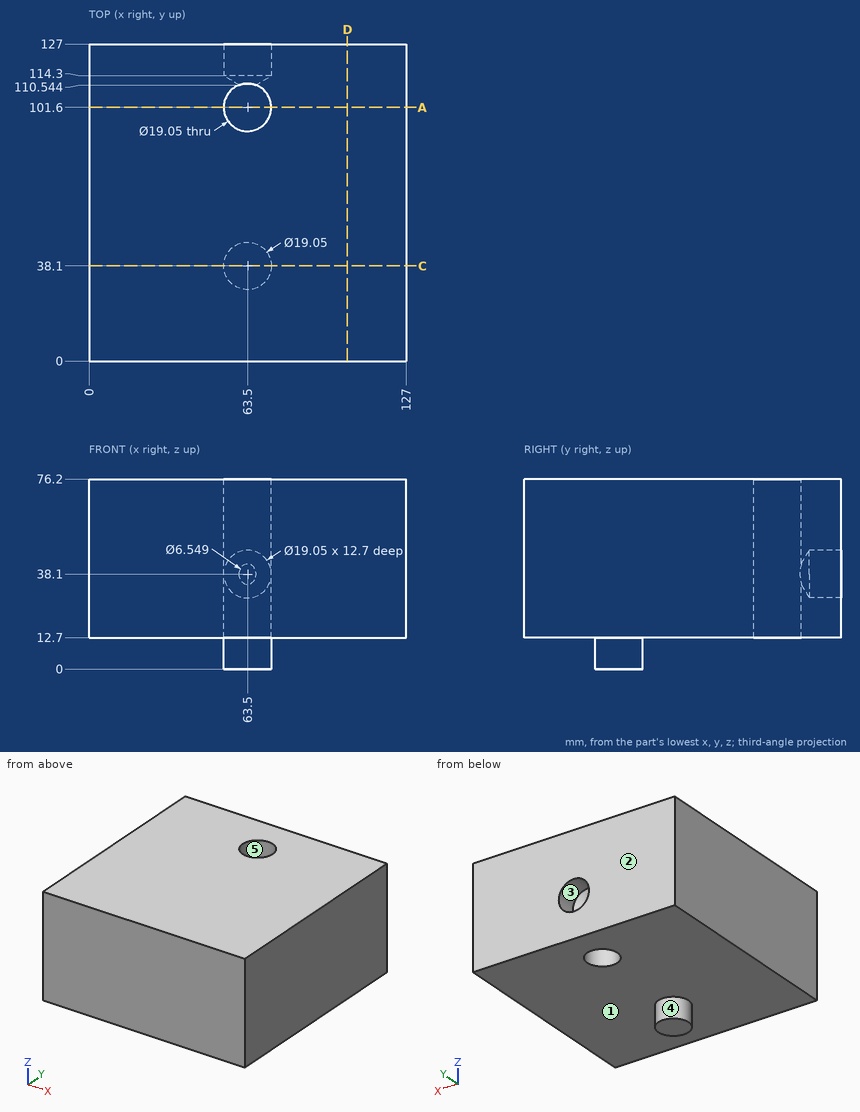
Part print with two shaded views. Sizes in mm from the minimum x, y, z corner. A direction names the side the tool comes from. Round coordinates to 2 decimals unless told otherwise and drop trailing zeros. Write each loop counter-clockwise with the first axis right and the second up, starting at its lowest first coordinate (ties: lowest second). Pieces come first, ordered by that corner, then holes. Notation, with made-up numbers: M 6.25,-34.75 L 29.25,-34.75 A12 ccw 29.25,-29.75 Z; hole C 73,46.5 d5. An arc over 180 degrees is marked long. Answer as CSV lines item,"result". Start each with the question number.
1) Mould opens along Z. For the marked faces 1, 2 and 3 say: +Z half, -Z half, draft (parallel to the pull), parting line (faces both ways), or undercut.
2) Band-saw the part on C-C (y = 38.1). List the corners of the cut face in (x, z) (1 decimal), then the cut area to 3 significant figures.
3) Drop flat-ended pins along their axis: pin 1 (17 mm diameter, centred on x = 63.5, z = 38.1, fed in from -Y); pin 2 (8 mm diameter, centred on x = 43.5, y = 86, fed in from -Z). Give the stop position or say it passes through.
4) Which spindle directions (+Z, -Z, +X, -X, +Y, -Y) get a long thin tool onto all of the face, cutting with end or side? Do the marked faces 4 and 5. Say none if no direction does.
5) Band-saw the part on A-A (y = 101.6). List the corners of the cut face in (x, z) (1 decimal).
6) Band-saw the part on D-D (x = 103.5). List the corners of the cut face in (y, z), then the cut area to 3 significant figures.
7) Drill centre lines: L1, parallel to X at y = 118.25, z = 38.1 (1 decimal); L2, parallel to Z at x = 63.5, y = 117.75 (1 decimal); L3, parallel to Z at x = 98, y = 117. Where is each one in solid material? Low to high.
Worked out:
1,face 1,"-Z half"
1,face 2,"draft"
1,face 3,"undercut"
2,outline,"M 0,12.7 L 54,12.7 L 54,0 L 73,0 L 73,12.7 L 127,12.7 L 127,76.2 L 0,76.2 Z"
2,area,"8,310 mm²"
3,pin 1,"y = 0"
3,pin 2,"z = 12.7"
4,face 4,"-Z"
4,face 5,"+Z, -Z"
5,outline,"M 0,12.7 L 54,12.7 L 54,76.2 L 0,76.2 Z; M 73,12.7 L 127,12.7 L 127,76.2 L 73,76.2 Z"
6,outline,"M 0,12.7 L 127,12.7 L 127,76.2 L 0,76.2 Z"
6,area,"8,060 mm²"
7,L1,"0 to 54, 73 to 127"
7,L2,"12.7 to 28.6, 47.6 to 76.2"
7,L3,"12.7 to 76.2"
